Read the model definition and answer for the solid it produces. Units are mm, in the model's axes. Give positions to 0.01 mm unless a question says otherwise; leave off trailing zeros. Loops run counter-clockwise (first coordinate to the right, second up) from the corner with the lowest first, then second, coordinate; pieces in that order, holes last. Notation, with made-up numbers: (88.25, 32.5) - (98.25, 32.5) arc R18 cw to (98.25, 48.5) - close; hole circle Ø11 at (33.25, -9.5). An arc over 180 degrees is marked (long way). Write item = value, one per line. Start each with the question number.
from build123d import *

# Parameters (mm, degrees)
SKETCH1_R           = 1.7
BOSS_EXTRUDE1_DEPTH = 1


with BuildPart() as part:
    # Sketch1 → Boss-Extrude1 (new body, symmetric)
    with BuildSketch(Plane.XY):
        with BuildLine():
            Line((35.2, 21.36), (30.8, 21.36))
            Line((30.8, 21.36), (30.8, -21.36))
            Line((30.8, -21.36), (35.2, -21.36))
            ThreePointArc((35.2, -21.36), (36.614213562, -20.774213562), (37.2, -19.36))
            Line((37.2, -19.36), (37.2, 19.36))
            ThreePointArc((37.2, 19.36), (36.614213562, 20.774213562), (35.2, 21.36))
        make_face()
        with Locations((34.16, -18.36)):
            Circle(SKETCH1_R, mode=Mode.SUBTRACT)
        with Locations((34.16, 18.36)):
            Circle(SKETCH1_R, mode=Mode.SUBTRACT)
    extrude(amount=BOSS_EXTRUDE1_DEPTH, both=True)


solid = part.part
1. A cutting plane is placed at D-D on y = -17.5. Give the vertices of the cut face in (x, z), and give its area (3 significant figures).
2. A cutting plane is placed at A-A on x = 34.16. Give the vertices of the cut face in (y, z), and give its area (3 significant figures).
3. Consider line 1 along Y through (x, z) = (34.16, 0.1); line 2 along Y through (x, z) = (35.25, -0.55); line 3 along Y through (x, z) = (37, 0.15). Determine where each line is inside the solid, lowest interval first. Write a range as [from, to].
4. Given P1, Ø3, axis at x = 34.16, y = 18.36, coming from the +Z side, flat-ended and moving along its own axis, determine where the tip first touches the part or whether it passes through.
5. A cutting plane is placed at C-C on z = -0.4. Give the vertices of the cut face in (x, y), and give its area (3 significant figures).
6. For a pull along X with two mould halves and no side action, classify faces 1 (the flat face through (33, -21.36, 0)), 2 (the cylindrical face through (36.6, -20.79, 0.01)), 3 (the flat face through (30.8, 0, 0)), 4 (the cylindrical face through (32.81, -19.39, -0.01)) as released by +X, released by -X, zero draft, split by the parting line, or undercut.
7. A cutting plane is placed at B-B on y = 18.36. Give the vertices of the cut face in (x, z), and give its area (3 significant figures).
Reply:
q1.outline = (30.8, -1) - (32.69, -1) - (32.69, 1) - (30.8, 1) - close; (35.63, -1) - (37.2, -1) - (37.2, 1) - (35.63, 1) - close
q1.area = 6.93 mm^2
q2.outline = (-21.36, -1) - (-20.06, -1) - (-20.06, 1) - (-21.36, 1) - close; (-16.66, -1) - (16.66, -1) - (16.66, 1) - (-16.66, 1) - close; (20.06, -1) - (21.36, -1) - (21.36, 1) - (20.06, 1) - close
q2.area = 71.8 mm^2
q3.line_1 = [-21.36, -20.06], [-16.66, 16.66], [20.06, 21.36]
q3.line_2 = [-21.36, -19.66], [-17.06, 17.06], [19.66, 21.36]
q3.line_3 = [-20.23, 20.23]
q4.P1 = through
q5.outline = (30.8, -21.36) - (35.2, -21.36) arc R2 ccw to (37.2, -19.36) - (37.2, 19.36) arc R2 ccw to (35.2, 21.36) - (30.8, 21.36) - close; hole circle Ø3.4 at (34.16, -18.36); hole circle Ø3.4 at (34.16, 18.36)
q5.area = 254 mm^2
q6.face_1 = zero draft
q6.face_2 = released by +X
q6.face_3 = released by -X
q6.face_4 = undercut
q7.outline = (30.8, -1) - (32.46, -1) - (32.46, 1) - (30.8, 1) - close; (35.86, -1) - (37.2, -1) - (37.2, 1) - (35.86, 1) - close
q7.area = 6.00 mm^2
